The figure shows three views and two pictorial views of one solid part (mm, origin at its lowest corner). Answer the questions. Coordinates: 2 decimals unless noted, no trailing zeros. Write each loop counter-clockwise with the first axis right and the second up, starting at its lowest first coordinate (ties: lowest second). Pieces come first, ordered by that corner, then holes. Notation, with made-up numbers: M 7,10.25 L 56,10.25 A10 cw 56,14.25 Z; hole C 84.25,-25.75 d2. An arc over 180 degrees is marked long. Write item = value, one per line. Start each with the question number.
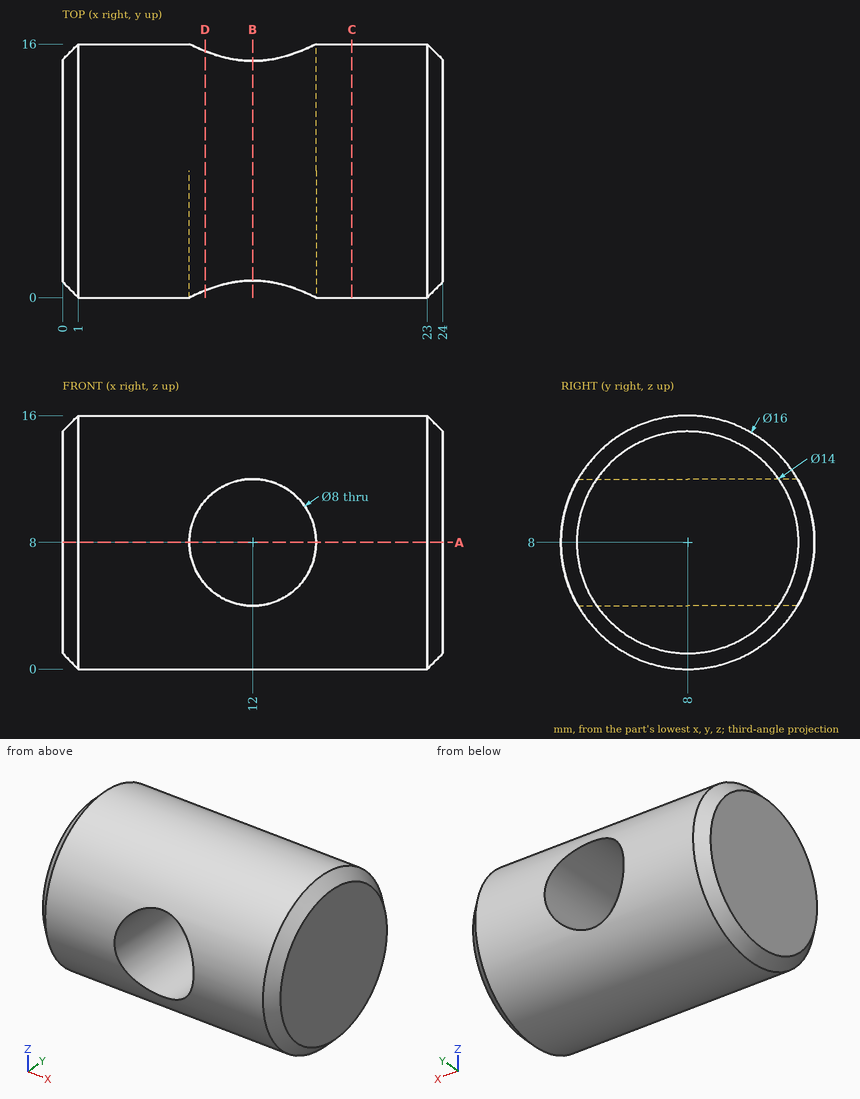
1. Each of these flat-tipped pins is pushed along its axis until it touches: pin 1 (8 mm diameter, centred on x = 19, z = 13.5, fed in from +Y); pin 2 (6.5 mm diameter, centred on x = 12, z = 8, fed in from +Y); pin 3 (4 mm diameter, centred on x = 10, y = 11.5, fed in from -Z); pin 4 (1 mm diameter, centred on x = 7.5, z = 13.5, fed in from +Y) (3 decimals). Where does it stop, or does it pass through?
2. The part is cut by section D-D, the plane x = 9. Write down the section's boundary in (y, z).
3. The part is cut by section B-B, the plane x = 12. Write down the section's boundary in (y, z), and give its area (3 significant figures).
4. Straight lines are drawn through the part: L1, parallel to X at y = 15, z = 5; L2, parallel to Z at x = 12, y = 14.25; L3, parallel to X at y = 3, z = 11.5. For each, find the intervals that lie inside material, in ascending order. Write a range as [from, to].
5. The part is cut by section A-A, the plane z = 8. Write down the section's boundary in (x, y), and give its area (3 significant figures).
6. The part is cut by section C-C, the plane x = 18.25. Write down the section's boundary in (y, z).
Solution:
q1.pin_1 = 15.86
q1.pin_2 = through
q1.pin_3 = 0.14
q1.pin_4 = 14.245
q2.outline = M 0.45,5.35 A8 ccw 15.55,5.35 Z; M 0.45,10.65 L 15.55,10.65 A8 ccw Z
q3.outline = M 1.07,4 A8 ccw 14.93,4 Z; M 1.07,12 L 14.93,12 A8 ccw Z
q3.area = 78.6 mm^2
q4.L1 = [0.62, 9.35], [14.65, 23.38]
q4.L2 = [3.01, 4], [12, 12.99]
q4.L3 = [0, 10.06], [13.94, 24]
q5.outline = M 0,1 L 1,0 L 8,0 L 8,16 L 1,16 L 0,15 Z; M 16,0 L 23,0 L 24,1 L 24,15 L 23,16 L 16,16 Z
q5.area = 254 mm^2
q6.outline = C 8,8 d16
